```python
from build123d import *

# Parameters (mm, degrees)
EXTRUDE_1_DEPTH           = 8
EXTRUDE_2_DEPTH           = 6
SKETCH_5_R                = 5
EXTRUDE_3_DEPTH           = 6
HOLE_WIZARD_1_D           = 5
HOLE_WIZARD_1_DEPTH       = 30
HOLE_WIZARD_1_CBORE_D     = 10
HOLE_WIZARD_1_CBORE_DEPTH = 4


with BuildPart() as part:
    # 草图3 → 凸台-拉伸1 (new body)
    with BuildSketch(Plane.XY):
        with BuildLine():
            Line((0, 0), (5, 0))
            ThreePointArc((5, 0), (9.784396345, -1.68635165), (12.453978369, -6))
            Line((12.453978369, -6), (8.243547108, -6))
            ThreePointArc((8.243547108, -6), (6.905295111, -4.540192237), (5, -4))
            Line((5, -4), (0, -4))
            Line((0, -4), (0, 0))
        make_face()
    extrude(amount=EXTRUDE_1_DEPTH)

    # 草图4 → 凸台-拉伸2 (add)
    with BuildSketch(Plane(origin=(0, 0, 0), x_dir=(1, 0, 0), z_dir=(0, 1, 0))):
        with BuildLine():
            Line((-0.255437353, 0), (0, 0))
            Line((0, 0), (0, -8))
            Line((0, -8), (-0.255437353, -8))
            ThreePointArc((-0.255437353, -8), (-13, -4), (-0.255437353, 0))
        make_face()
    extrude(amount=-EXTRUDE_2_DEPTH)

    # 草图5 → 凸台-拉伸3 (add)
    with BuildSketch(Plane.XZ.offset(6)):
        with Locations((-6, 4)):
            Circle(SKETCH_5_R)
    extrude(amount=EXTRUDE_3_DEPTH)

    # 孔1
    with Locations(Plane(origin=(-6, 0, 4), x_dir=(0, 0, 1), z_dir=(0, 1, 0))):
        with Locations((0, 0)):
            CounterBoreHole(HOLE_WIZARD_1_D / 2, HOLE_WIZARD_1_CBORE_D / 2, HOLE_WIZARD_1_CBORE_DEPTH, depth=HOLE_WIZARD_1_DEPTH)


solid = part.part
```
Input: part model. Units: mm. Frame: model coordinates. A direction names the side the tool comes from. Coordinates: 2 decimals unless noted, no trailing zeros. Write each loop counter-clockwise with the first axis right and the second up, starting at its lowest first coordinate (ties: lowest second). Pieces come first, ordered by that corner, then holes.
1) Material intervals for line 1 along X through (y, z) = (-4.5, 4); line 2 along Y through (x, z) = (-2.5, 0.25); line 3 along Y through (x, z) = (-5, 8.75), sorted ascending.
2) Section D-D on x = -2.75. Output: boundary loops of the cut face in (y, z), and give its area (3 significant figures).
3) Pin query (flat end, axial travel): pin 1 Ø3 at (x, y) = (3, -4) entering from +Z; pin 2 Ø3 at (x, z) = (-6.5, 3) entering from +Y; pin 3 Ø4 at (x, y) = (-0.5, -4) entering from -Z. Return the tip coordinate at first contact, or that it passes through.
4) Set-up query: faces 1 (the flat face through (-8, -4, 6)), 2 (the flat face through (6, -3, 8)), 3 (the flat face through (3, -4, 4)). Return all of +Z, -Z, +X, -X, +Y, -Y with unobstructed straight access to the full face (end or side cutting, diameter ignored); none if empty.
5) Section A-A on x = -6. Output: boundary loops of the cut face in (y, z), and give its area (3 significant figures).
6) Section B-B on y = -5. Output: boundary loops of the cut face in (x, z).
7) Section C-C on z = 4. Output: boundary loops of the cut face in (x, y), and give its area (3 significant figures).
8) Mould query, pull axis Z, two halves, no side actions, for faces 4 (the cylindrical face through (-7.08, -8.96, -0.88)), 5 (the flat face through (6, -3, 0)), 6 (the cylindrical face through (-9, -2, 0)), 7 (the flat face through (10, -6, 4)). Classes: pulls with the +Z half, pulls with the -Z half, needs draft (parallel to the pull), parting line crosses it, or undercut.
Check result:
1. line 1: x = -13 to -8.5, -3.5 to 0, 6.84 to 11.96
1. line 2: y = -6 to 0
1. line 3: y = -12 to -4
2. outline: (-12, 0.2) - (-6, 0.2) - (-6, -2.2) - (0, -2.2) - (0, 0.2) - (-4, 0.2) - (-4, 7.8) - (0, 7.8) - (0, 10.2) - (-6, 10.2) - (-6, 7.8) - (-12, 7.8) - close
2. area: 89.6 mm2
3. pin 1: stops at z = 8
3. pin 2: stops at y = -4
3. pin 3: stops at z = -2.06
4. face 1: +Y
4. face 2: +Z, +X, +Y, -Y
4. face 3: +Z, -Z, -Y
5. outline: (-12, -1) - (-6, -1) - (-6, -3) - (0, -3) - (0, -1) - (-4, -1) - (-4, 1.5) - (-12, 1.5) - close; (-12, 6.5) - (-4, 6.5) - (-4, 9) - (0, 9) - (0, 11) - (-6, 11) - (-6, 9) - (-12, 9) - close
5. area: 64.0 mm2
6. outline: (-0.26, 0) - (0, 0) - (0, 8) - (-0.26, 8) arc R7 ccw (long way) to start; (7.5, 0) - (12.16, 0) - (12.16, 8) - (7.5, 8) - close; hole circle Ø5 at (-6, 4)
7. outline: (-13, -6) - (-11, -6) - (-11, -12) - (-8.5, -12) - (-8.5, -4) - (-11, -4) - (-11, 0) - (-13, 0) - close; (-3.5, -12) - (-1, -12) - (-1, -6) - (0, -6) - (0, -4) - (5, -4) arc R3.63 cw to (8.24, -6) - (12.45, -6) arc R7.63 ccw to (5, 0) - (-1, 0) - (-1, -4) - (-3.5, -4) - close
7. area: 107 mm2
8. face 4: parting line crosses it
8. face 5: pulls with the -Z half
8. face 6: undercut
8. face 7: needs draft
